Source: three-view drawing plus pictorial views. Frame: mm from the lowest corner of the part. Coordinates: 2 decimals unless noted, no trailing zeros. Loops run counter-clockwise (first coordinate to the right, second up) from the corner with the lowest first, then second, coordinate; pieces in that order, holes last. Notation, with made-up numbers: (-20.75, -5.75) - (37.25, -5.75) arc R30 ccw to (37.25, 18.25) - close; hole circle Ø3 at (74.25, 77). An arc over 180 degrees is marked (long way). Return JSON: item names as keys, results as strings.
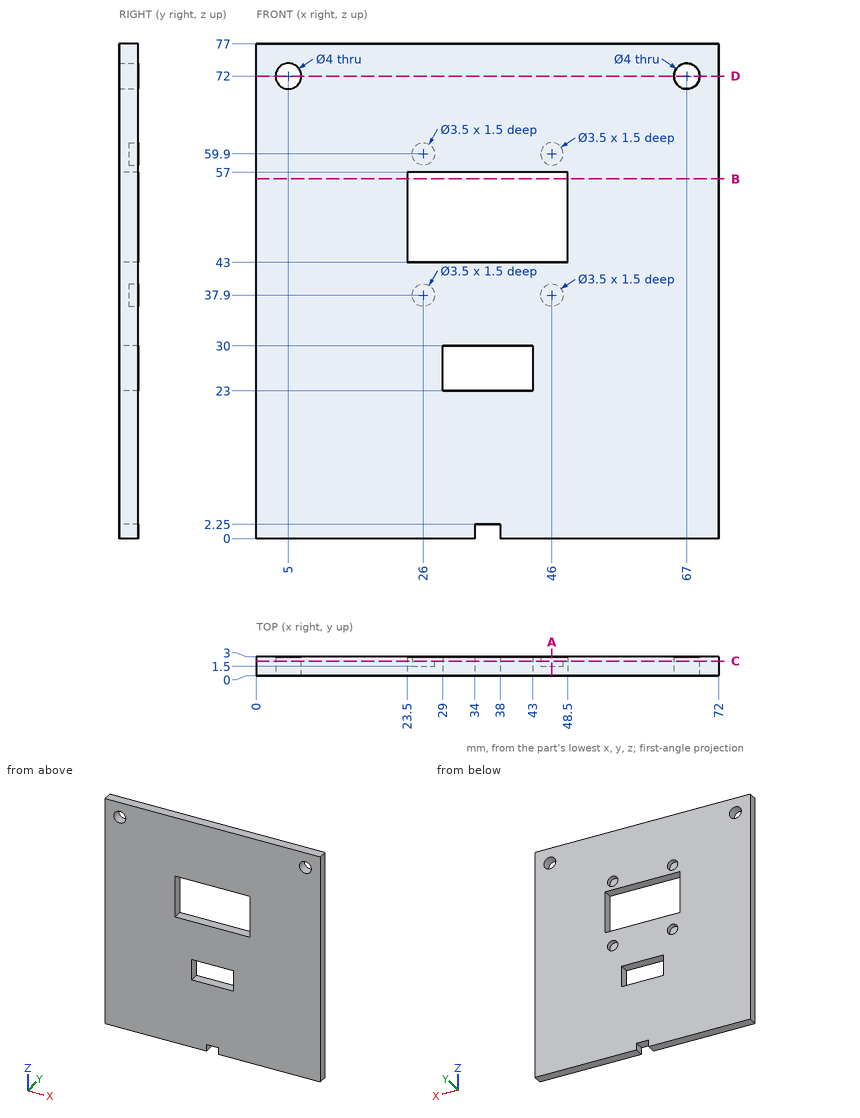
Item 1: First-contact query: pin 1 Ø3 at (x, z) = (26, 60.5) entering from +Y; pin 2 Ø1.5 at (x, y) = (35.5, 2) entering from -Z. Flat tips, straight axial feed; report the tip coordinate or a pass-through.
Worked out:
{"pin 1": "y = 3", "pin 2": "z = 2.25"}
Item 2: Section query B-B, the plane z = 56. Return loops of the section in (x, y), and give its area (3 significant figures).
Worked out:
{"outline": "(0, 0) - (23.5, 0) - (23.5, 3) - (0, 3) - close; (48.5, 0) - (72, 0) - (72, 3) - (48.5, 3) - close", "area": "141 mm^2"}
Item 3: Section query C-C, the plane y = 2.3. Count the separate pieces of the cut face and the enclosed holes in it, and give its area (3 significant figures).
Worked out:
{"separate pieces": "1", "enclosed holes": "8", "area": "5,020 mm^2"}
Item 4: Section query A-A, the plane x = 46. Return loops of the section in (y, z).
Worked out:
{"outline": "(0, 0) - (3, 0) - (3, 36.15) - (1.5, 36.15) - (1.5, 39.65) - (3, 39.65) - (3, 43) - (0, 43) - close; (0, 57) - (3, 57) - (3, 58.15) - (1.5, 58.15) - (1.5, 61.65) - (3, 61.65) - (3, 77) - (0, 77) - close"}
Item 5: Ray query, probe 1 along Z at (x, y) = (46, 2.05); probe 2 along X at (y, z) = (2.2, 72); probe 3 along Z at (x, y) = (35.5, 0.4). Return the intervals inside material, ascending. Write a range as from..to.
Worked out:
{"probe 1": "0..36.15, 39.65..43, 57..58.15, 61.65..77", "probe 2": "0..3, 7..65, 69..72", "probe 3": "2.25..23, 30..43, 57..77"}
Item 6: Section query D-D, the plane z = 72. Return loops of the section in (x, y).
Worked out:
{"outline": "(0, 0) - (3, 0) - (3, 3) - (0, 3) - close; (7, 0) - (65, 0) - (65, 3) - (7, 3) - close; (69, 0) - (72, 0) - (72, 3) - (69, 3) - close"}
